from build123d import *

# Parameters (mm, degrees)
F0_W     = 50
F0_H     = 55
F1_DEPTH = 50
F2_T     = -2.54
F3_W     = 11
F3_H     = 11
F4_DEPTH = 10
F5_W     = 11
F5_H     = 11
F6_DEPTH = 10


with BuildPart() as f1:
    # F0 (on Front) → F1 (new body)
    with BuildSketch(Plane.XZ):
        Rectangle(F0_W, F0_H)
    extrude(amount=-F1_DEPTH)

    # F2
    f2_openings = [f1.faces().sort_by_distance(p)[0] for p in [
        (0, 25, -27.5),
    ]]
    offset(amount=F2_T, openings=f2_openings)

    # F3 (on face) → F4 (cut)
    with BuildSketch(Plane(origin=(-25, 0, 0), x_dir=(0, -1, 0), z_dir=(-1, 0, 0))):
        with Locations((-32.5, 3)):
            Rectangle(F3_W, F3_H)
    extrude(amount=-F4_DEPTH, mode=Mode.SUBTRACT)

    # F5 (on face) → F6 (cut)
    with BuildSketch(Plane.YZ.offset(25)):
        with Locations((17.5, 3)):
            Rectangle(F5_W, F5_H)
    extrude(amount=-F6_DEPTH, mode=Mode.SUBTRACT)


solid = f1.part
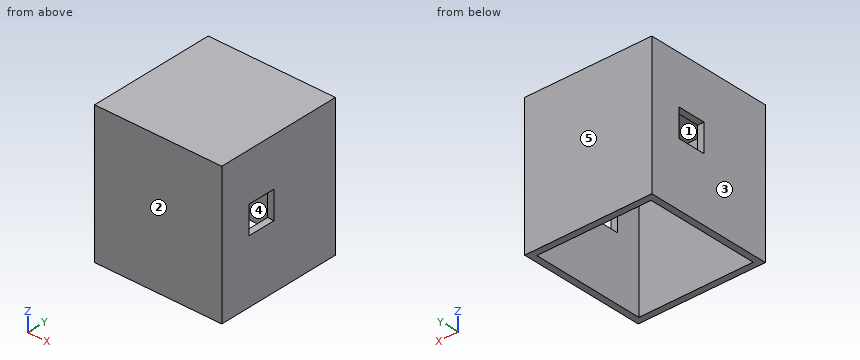
The listing builds one solid part. Answer for the finished solid, in the listing's coordinates (mm). Face numbers are marked on the shaded views. A direction names the side the tool comes from. Round coordinates to 2 decimals unless told otherwise and drop trailing zeros. Order: outer loops, then holes, each group sorted by start corner. A loop starts at its lowest first (then second) coordinate and runs counter-clockwise, first axis right, second up. Notation, with made-up numbers: (79.25, 66.25) -> (138.25, 66.25) arc R26 cw to (138.25, 105.25) -> close; hole circle Ø5 at (57, 23.5). An arc over 180 degrees is marked (long way). Write each question's results on one line, items separated by ' | '. Start each with the question number.
Q1. Find section C-C (x = -0.5). Determine the outline of the cut face in (y, z).
Q2. Find section B-B (y = 22). Determine the outline of the cut face in (x, z), then the cut area to 3 significant figures.
Q3. Which of the six approach directions +Z, -Z, +X, -X, +Y, -Y give full straight-line access (tool end or side, diameter ignored) to the marked faces 1 and 2?
Q4. Find section A-A (z = 20). Determine the outline of the cut face in (x, y).
Q5. Straight lines are drawn through the part: probe 1 along Y at (x, z) = (-15, -3.5); probe 2 along X at (y, z) = (35.5, 17); probe 3 along Z at (x, y) = (14, 21). For each, find the intervals that lie inside material, in ascending order. Write a range as from..to.
Q6. This flat-tipped pin is pushed along its axis until it touches: pin 1 (4 mm diameter, centred on x = 2, y = 14, fed in from -Z). Where does it stop, or does it pass through?
Q7. The mould has two halves that part along X. Classify the marked faces 3, 4 and 5: pulls with the +X half, pulls with the -X half, needs draft (parallel to the pull), parting line crosses it, or undercut.
Worked answers:
1) outline: (0, -27.5) -> (2.54, -27.5) -> (2.54, 24.96) -> (47.46, 24.96) -> (47.46, -27.5) -> (50, -27.5) -> (50, 27.5) -> (0, 27.5) -> close
2) outline: (-25, -27.5) -> (-22.46, -27.5) -> (-22.46, 24.96) -> (22.46, 24.96) -> (22.46, 8.5) -> (25, 8.5) -> (25, 27.5) -> (-25, 27.5) -> close; (22.46, -27.5) -> (25, -27.5) -> (25, -2.5) -> (22.46, -2.5) -> close | area: 366 mm2
3) face 1: -Z | face 2: +Z, -Z, +X, -X, -Y
4) outline: (-25, 0) -> (25, 0) -> (25, 50) -> (-25, 50) -> close; hole (-22.46, 2.54) -> (22.46, 2.54) -> (22.46, 47.46) -> (-22.46, 47.46) -> close
5) probe 1: y = 0..2.54, 47.46..50 | probe 2: x = -25..-22.46, 22.46..25 | probe 3: z = 24.96..27.5
6) pin 1: stops at z = 24.96
7) face 3: pulls with the -X half | face 4: undercut | face 5: needs draft
